```python
from build123d import *

# Parameters (mm, degrees)
F0_W     = 190.5
F0_H     = 76.2
F1_DEPTH = 6.35
F3_D     = 6.5278
F4_W     = 38.1
F4_H     = 38.1
F4_W_2   = 28.575
F4_H_2   = 28.575
F5_DEPTH = 50.8
F6_R     = 3.175
F7_R     = 6.35
F8_DEPTH = 38.1


# Not quite as in the source:
# - a feature names something its author has since deleted; it is built from what else it names


with BuildPart() as f1:
    # F0 (on Top) → F1 (new body, symmetric)
    with BuildSketch(Plane.XY):
        Rectangle(F0_W, F0_H)
    extrude(amount=F1_DEPTH, both=True)

    # F3 (through all)
    with Locations(Plane(origin=(0, 0, -6.35), x_dir=(1, 0, 0), z_dir=(0, 0, -1))):
        with Locations((-76.2, -25.4), (-25.4, -25.4), (-76.2, 25.4), (-25.4, 25.4), (25.4, 25.4), (25.4, -25.4), (76.2, -25.4), (76.2, 25.4)):
            Hole(F3_D / 2)

    # F4 (on face) → F5 (join)
    with BuildSketch(Plane.XY.offset(6.35)):
        Rectangle(F4_W, F4_H)
        Rectangle(F4_W_2, F4_H_2, mode=Mode.SUBTRACT)
    extrude(amount=F5_DEPTH)

    # F6
    f6_edges = [f1.edges().sort_by_distance(p)[0] for p in [
        (-19.05, -19.05, 31.75),
        (19.05, -19.05, 31.75),
        (-14.2875, 14.2875, 31.75),
        (14.2875, 14.2875, 31.75),
        (-14.2875, -14.2875, 31.75),
        (14.2875, -14.2875, 31.75),
        (-19.05, 19.05, 31.75),
        (19.05, 19.05, 31.75),
    ]]
    fillet(f6_edges, radius=F6_R)

    # F7 (on face) → F8 (cut, through all)
    with BuildSketch(Plane.XZ.offset(19.05)):
        with Locations((0, 19.05)):
            Circle(F7_R)
    extrude(amount=-F8_DEPTH, mode=Mode.SUBTRACT)


solid = f1.part
```
Part model, mm, in its own coordinate system. A direction names the side the tool comes from. Round coordinates to 2 decimals unless told otherwise and drop trailing zeros. Loops run counter-clockwise (first coordinate to the right, second up) from the corner with the lowest first, then second, coordinate; pieces in that order, holes last.
Item 1: Mould opens along Y. For faces 4 (the face through (73.087, -26.38, 0.089)), 5 (the face through (3.414, 16.635, 24.404)), 6 (the face through (0, -19.05, 31)) say: +Y half, -Y half, draft (parallel to the pull), parting line (faces both ways), or undercut.
Item 2: Drop flat-ended pins along their axis: P1, Ø11, axis at y = -2.5, z = 37, coming from the -X side; P2, Ø14.5, axis at x = 0, z = 19.05, coming from the -Y side; P3, Ø1, axis at y = 5, z = 12, coming from the +X side. Give the stop position or say it passes through.
Item 3: Cut at B-B, the plane x = 0. Give the cut face in (y, z).
Item 4: Drill centre lines: line 1 (Y direction, x = -76, z = 0); line 2 (X direction, y = -25, z = 0); line 3 (X direction, y = 25.4, z = 3.5). Where is each one in solid material? Low to high.
Item 5: Cut at C-C, the plane z = 3.5. State how many separate pieces and enclosed holes the cut face has, then the cut area to 3 significant figures.
Item 6: Cut at A-A, the plane y = -25.4. Give the cut face in (x, z), then the cut area to 3 significant figures.
Item 7: 3-axis set-ups, long thin cutter, end or side, ignore diameter. For faces 1 (the face through (-17, 0, 57.15)), 2 (the face through (-14.288, 0, 31)), 3 (the face through (0, 19.05, 31)): which of +Z, -Z, +X, -X, +Y, -Y reach the whole face in a straight line?
A:
1. face 4: undercut
1. face 5: draft
1. face 6: -Y half
2. P1: stops at x = -19.05
2. P2: stops at y = -19.05
2. P3: stops at x = 19.05
3. outline: (-38.1, -6.35) - (38.1, -6.35) - (38.1, 6.35) - (19.05, 6.35) - (19.05, 12.7) - (14.29, 12.7) - (14.29, 6.35) - (-14.29, 6.35) - (-14.29, 12.7) - (-19.05, 12.7) - (-19.05, 6.35) - (-38.1, 6.35) - close; (-19.05, 25.4) - (-14.29, 25.4) - (-14.29, 57.15) - (-19.05, 57.15) - close; (14.29, 25.4) - (19.05, 25.4) - (19.05, 57.15) - (14.29, 57.15) - close
4. line 1: y = -38.1 to -28.66, -22.14 to 22.14, 28.66 to 38.1
4. line 2: x = -95.25 to -79.44, -72.96 to -28.64, -22.16 to 22.16, 28.64 to 72.96, 79.44 to 95.25
4. line 3: x = -95.25 to -79.46, -72.94 to -28.66, -22.14 to 22.14, 28.66 to 72.94, 79.46 to 95.25
5. separate pieces: 1
5. enclosed holes: 8
5. area: 14,200 mm2
6. outline: (-95.25, -6.35) - (-79.46, -6.35) - (-79.46, 6.35) - (-95.25, 6.35) - close; (-72.94, -6.35) - (-28.66, -6.35) - (-28.66, 6.35) - (-72.94, 6.35) - close; (-22.14, -6.35) - (22.14, -6.35) - (22.14, 6.35) - (-22.14, 6.35) - close; (28.66, -6.35) - (72.94, -6.35) - (72.94, 6.35) - (28.66, 6.35) - close; (79.46, -6.35) - (95.25, -6.35) - (95.25, 6.35) - (79.46, 6.35) - close
6. area: 2,090 mm2
7. face 1: +Z, +X, -X, +Y, -Y
7. face 2: +Z
7. face 3: +Z, +X, -X, +Y
